The listing builds one solid part. Answer for the finished solid, in the listing's coordinates (mm). A direction names the side the tool comes from. Round coordinates to 2 decimals unless told otherwise and drop trailing zeros. Write each loop counter-clockwise with the first axis right and the second up, starting at its lowest first coordinate (ties: lowest second). Pieces come first, ordered by that corner, then holes. Notation, with made-up numbers: (74, -10.5) - (101, -10.5) arc R36 ccw to (101, 24.5) - close; hole circle Ø5 at (22, 59.5). An arc over 180 degrees is marked (long way). Return JSON: item names as keys, results as strings. Group by question number.
(1) Which of the six approach directions +Z, -Z, +X, -X, +Y, -Y give full straight-line access (tool end or side, diameter ignored) to faces 1 (the cylindrical face through (-86.056, -1.521, -44.76)), 2 (the flat face through (81.9, -3, 52.3))?
(2) Section C-C, the plane y = -1 is taken. Write down the section's boundary in (x, z).
(3) Each of these flat-tipped pins is pushed along its axis until it touches: pin 1 (1.5 mm diameter, centred on x = 13.5, y = 0.5, fed in from +Z); pin 2 (3.5 mm diameter, centred on x = -18.56, z = -11.94, fed in from -Y); pin 3 (3 mm diameter, centred on x = 39.94, z = -75.03, fed in from -Y); pin 4 (3 mm diameter, centred on y = 1, z = -67.5, fed in from +X). Where does it stop, or does it pass through?
(4) Determine the mould class of faces 3 (the flat face through (1, 0, -1)), 4 (the flat face through (1, 3, -1)) for opening direction Z: +Z half, -Z half, draft (parallel to the pull), parting line (faces both ways), or undercut.
(5) Section B-B, the plane x = 0 is taken. Write down the section's boundary in (y, z), then the cut area to 3 significant figures.
(6) Find the intervals of material crossed by line 1 along X through (y, z) = (1.4, 11.94); line 2 along Z through (x, y) = (40.5, 2.25); line 3 along Y through (x, z) = (25, -16), in increasing order. Write a range as [from, to].
(7) Section A-A, the plane z = 0 is taken. Write down the section's boundary in (x, y).
```python
from build123d import *

# Parameters (mm, degrees)
SKETCH_1_R          = 100
EXTRUDE_1_DEPTH     = 3
SKETCH_5_R          = 2
CUT_EXTRUDE_3_DEPTH = 10
SKETCH_6_R          = 1.5
CUT_EXTRUDE_4_DEPTH = 10
SKETCH_7_RX         = 14.914689971
SKETCH_7_RY         = 8.256346234
CUT_EXTRUDE_5_DEPTH = 10
EXTRUDE_START       = 3
SKETCH_9_R          = 100
SKETCH_9_R_2        = 97
EXTRUDE_3_DEPTH     = 3


with BuildPart() as part:
    # Эскиз1 → Бобышка-Вытянуть1 (new body)
    with BuildSketch(Plane(origin=(0, 0, 0), x_dir=(1, 0, 0), z_dir=(0, 1, 0))):
        with Locations(Location((0, 0, 0), (0, 0, 270))):
            Circle(SKETCH_1_R)
    extrude(amount=EXTRUDE_1_DEPTH)

    # Эскиз5 → Вырез-Вытянуть3 (cut)
    with BuildSketch(Plane(origin=(0, 3, 0), x_dir=(1, 0, 0), z_dir=(0, 1, 0))):
        with Locations(Location((39.936936383, -75.033599889, 0), (0, 0, 270))):
            Circle(SKETCH_5_R)
        with Locations(Location((39.936936383, 75.033599889, 0), (0, 0, 270))):
            Circle(SKETCH_5_R)
        with Locations(Location((-65, 54.772255751, 0), (0, 0, 270))):
            Circle(SKETCH_5_R)
        with Locations(Location((-65, -54.772255751, 0), (0, 0, 270))):
            Circle(SKETCH_5_R)
    extrude(amount=-CUT_EXTRUDE_3_DEPTH, mode=Mode.SUBTRACT)

    # Эскиз6 → Вырез-Вытянуть4 (cut)
    with BuildSketch(Plane(origin=(0, 3, 0), x_dir=(1, 0, 0), z_dir=(0, 1, 0))):
        with Locations(Location((-65.064398668, 11.94, 0), (0, 0, 270))):
            Circle(SKETCH_6_R)
        with Locations(Location((-18.564398668, 11.94, 0), (0, 0, 270))):
            Circle(SKETCH_6_R)
        with Locations(Location((-18.564398668, -11.94, 0), (0, 0, 270))):
            Circle(SKETCH_6_R)
        with Locations(Location((-65.064398668, -11.94, 0), (0, 0, 270))):
            Circle(SKETCH_6_R)
        with Locations(Location((34.209802243, -10.340313566, 0), (0, 0, 270))):
            Circle(SKETCH_6_R)
        with Locations(Location((34.82871581, 11.665691446, 0), (0, 0, 270))):
            Circle(SKETCH_6_R)
        with Locations(Location((-45.249923126, 13.677319461, 0), (0, 0, 270))):
            Circle(SKETCH_6_R)
        with Locations(Location((-44.893210092, -15.036739793, 0), (0, 0, 270))):
            Circle(SKETCH_6_R)
    extrude(amount=-CUT_EXTRUDE_4_DEPTH, mode=Mode.SUBTRACT)

    # Эскиз7 → Вырез-Вытянуть5 (cut)
    with BuildSketch(Plane(origin=(0, 3, 0), x_dir=(1, 0, 0), z_dir=(0, 1, 0))):
        with Locations((-27.965043695, 48.472742405)):
            Ellipse(SKETCH_7_RX, SKETCH_7_RY)
        with Locations((-27.965043695, -48.472742405)):
            Ellipse(SKETCH_7_RX, SKETCH_7_RY)
    extrude(amount=-CUT_EXTRUDE_5_DEPTH, mode=Mode.SUBTRACT)

    # Эскиз9 → Бобышка-Вытянуть3 (add)
    with BuildSketch(Plane.XZ.offset(EXTRUDE_START)):
        with Locations(Location((0, 0, 0), (0, 0, 270))):
            Circle(SKETCH_9_R)
        with Locations(Location((0, 0, 0), (0, 0, 270))):
            Circle(SKETCH_9_R_2, mode=Mode.SUBTRACT)
    extrude(amount=-EXTRUDE_3_DEPTH)


solid = part.part
```
Working result:
{
 "1": {"face 1": "-Y", "face 2": "+Z, -Z, +X, -X, -Y"},
 "2": {"outline": "circle Ø200 at (0, 0); hole circle Ø194 at (0, 0)"},
 "3": {"pin 1": "stops at z = 99.18", "pin 2": "stops at y = 0", "pin 3": "passes through", "pin 4": "stops at x = 75.13"},
 "4": {"face 3": "undercut", "face 4": "draft"},
 "5": {"outline": "(-3, -100) - (3, -100) - (3, 100) - (-3, 100) - (-3, 97) - (0, 97) - (0, -97) - (-3, -97) - close", "area": "618 mm^2"},
 "6": {"line 1": "x = [-99.28, -66.56], [-63.56, -20.06], [-17.06, 99.28]", "line 2": "z = [-91.43, -76.95], [-73.11, 73.11], [76.95, 91.43]", "line 3": "y = [0, 3]"},
 "7": {"outline": "(-100, -3) - (-97, -3) - (-97, 0) - (97, 0) - (97, -3) - (100, -3) - (100, 3) - (-100, 3) - close"}
}
